from build123d import *

# Parameters (mm, degrees)
SKETCH35_R          = 1.5875
SKETCH35_R_2        = 55.372
BOSS_EXTRUDE5_DEPTH = 3.175


with BuildPart() as part:
    # Sketch35 → Boss-Extrude5 (new body)
    with BuildSketch(Plane(origin=(0, 0, 0), x_dir=(1, 0, 0), z_dir=(0, 1, 0))):
        with BuildLine():
            ThreePointArc((72.63160158, -196.735304264), (79.763343901, -189.694281524), (72.63160158, -182.653258784))
            ThreePointArc((72.63160158, -182.653258784), (71.923524594, -182.763416409), (71.274394231, -183.066957991))
            ThreePointArc((71.274394231, -183.066957991), (62.061766366, -186.749902585), (52.140854077, -186.639937081))
            ThreePointArc((52.140854077, -186.639937081), (49.212807322, -185.841233605), (46.400330688, -184.700461837))
            ThreePointArc((46.400330688, -184.700461837), (40.308522411, -162.14266409), (26.470306292, -143.315339746))
            ThreePointArc((26.470306292, -143.315339746), (2.051929923, -129.089326239), (-26.120702924, -126.866867398))
            ThreePointArc((-26.120702924, -126.866867398), (-27.858708089, -124.378751024), (-29.2889381, -121.701844758))
            ThreePointArc((-29.2889381, -121.701844758), (-31.603757208, -112.05414008), (-30.063154281, -102.252959759))
            ThreePointArc((-30.063154281, -102.252959759), (-29.911668214, -101.552560093), (-29.961834423, -100.837723697))
            ThreePointArc((-29.961834423, -100.837723697), (-38.413285984, -95.451564003), (-43.690813622, -103.971273609))
            ThreePointArc((-43.690813622, -103.971273609), (-43.425855926, -104.63708525), (-42.98547967, -105.202396203))
            ThreePointArc((-42.98547967, -105.202396203), (-37.34487163, -113.364511982), (-35.244469401, -123.061155914))
            ThreePointArc((-35.244469401, -123.061155914), (-35.371596014, -126.093518667), (-35.857931325, -129.089326239))
            ThreePointArc((-35.857931325, -129.089326239), (-74.114523813, -162.14266409), (-76.104068675, -212.661291576))
            ThreePointArc((-76.104068675, -212.661291576), (-78.143060244, -214.909379303), (-80.434594764, -216.899418143))
            ThreePointArc((-80.434594764, -216.899418143), (-89.325315633, -221.303016159), (-99.223576302, -221.982007162))
            ThreePointArc((-99.223576302, -221.982007162), (-99.940124308, -221.990172755), (-100.625875231, -222.198147255))
            ThreePointArc((-100.625875231, -222.198147255), (-103.996367762, -231.636236566), (-94.515904683, -234.885631829))
            ThreePointArc((-94.515904683, -234.885631829), (-93.925744965, -234.479160148), (-93.472600473, -233.924031523))
            ThreePointArc((-93.472600473, -233.924031523), (-86.770279347, -226.608603676), (-77.784133989, -222.403156653))
            ThreePointArc((-77.784133989, -222.403156653), (-74.799510568, -221.852331744), (-71.770594359, -221.659843715))
            ThreePointArc((-71.770594359, -221.659843715), (-52.467656797, -242.300414596), (-26.120702924, -252.52169565))
            ThreePointArc((-26.120702924, -252.52169565), (-2.772921395, -251.602203947), (18.661655395, -242.300414596))
            ThreePointArc((18.661655395, -242.300414596), (21.307097177, -243.788037808), (23.75715599, -245.579293472))
            ThreePointArc((23.75715599, -245.579293472), (30.028718121, -253.267212663), (32.893255611, -262.766213559))
            ThreePointArc((32.893255611, -262.766213559), (33.060663407, -263.462979195), (33.416017488, -264.085258231))
            ThreePointArc((33.416017488, -264.085258231), (43.367479341, -265.271073029), (44.425803982, -255.305246485))
            ThreePointArc((44.425803982, -255.305246485), (43.898200503, -254.82033176), (43.256155975, -254.502076287))
            ThreePointArc((43.256155975, -254.502076287), (34.632734421, -249.595632182), (28.533121278, -241.770588249))
            ThreePointArc((28.533121278, -241.770588249), (27.331965509, -238.983365642), (26.470306292, -236.073223302))
            ThreePointArc((26.470306292, -236.073223302), (40.308522411, -217.245898958), (46.400330688, -194.68810121))
            ThreePointArc((46.400330688, -194.68810121), (49.212807322, -193.547329442), (52.140854077, -192.748625967))
            ThreePointArc((52.140854077, -192.748625967), (62.061766366, -192.638660462), (71.274394231, -196.321605056))
            ThreePointArc((71.274394231, -196.321605056), (71.923524594, -196.625146639), (72.63160158, -196.735304264))
        make_face()
        with Locations(Location((72.72174416, -189.694281524, 0), (0, 0, 270))):
            Circle(SKETCH35_R, mode=Mode.SUBTRACT)
        with Locations(Location((-16.903000701, -189.694281524, 0), (0, 0, 270))):
            Circle(SKETCH35_R_2, mode=Mode.SUBTRACT)
        with Locations(Location((-97.652105615, -228.581000942, 0), (0, 0, 270))):
            Circle(SKETCH35_R, mode=Mode.SUBTRACT)
        with Locations(Location((-36.846382633, -102.316616136, 0), (0, 0, 270))):
            Circle(SKETCH35_R, mode=Mode.SUBTRACT)
        with Locations(Location((38.977113714, -259.765728664, 0), (0, 0, 270))):
            Circle(SKETCH35_R, mode=Mode.SUBTRACT)
    extrude(amount=BOSS_EXTRUDE5_DEPTH)


solid = part.part
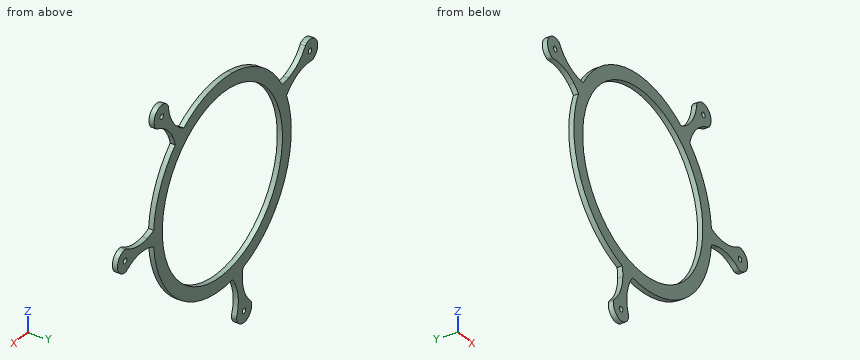
Build history of the part. All positions in model axes, mm. Round coordinates to 2 decimals unless told otherwise and drop trailing zeros. Order: outer loops, then holes, each group sorted by start corner. A loop starts at its lowest first (then second) coordinate and runs counter-clockwise, first axis right, second up. Notation, with made-up numbers: M 66,-26.75 L 115,-26.75 A9 cw 115,-14.75 Z; hole C 28.25,-9.75 d6. An arc over 180 degrees is marked long. Use CSV: the item, a comma, the result in double quotes. Start each with the question number.
(1) Cut at B-B on z = 179.5. List the corners of the cut face in (x, y) (1 decimal).
(2) Cut at C-C on y = 1. State how many separate pieces and enclosed holes the cut face has, then the cut area to 3 significant figures.
(3) Flat gauge pins, fed straight in: P1, Ø1, axis at x = 38.5, y = 2, coming from the -Z side; P2, Ø1.5, axis at y = 2, z = 166.5, coming from the +X side; P3, Ø1, axis at y = 1.5, z = 232.5, coming from the +X side. Where does each tip first touch, or does it go through?
(4) Cut at A-A on x = 8.5. List the corners of the cut face in (y, z) (3 decimals), then the cut area to 3 significant figures.
(5) Drill centre lines: probe 1 along X at (y, z) = (0.3, 190); probe 2 along X at (y, z) = (0.6, 195); probe 3 along Z at (x, y) = (34.5, 2.2). Where is each one in solid material? Low to high.
(6) Cut at D-D on z = 114. List the corners of the cut face in (x, y) (3 decimals).
Findings:
1,outline,"M -79.6,0 L -71.3,0 L -71.3,3.2 L -79.6,3.2 Z; M 37.5,0 L 45.8,0 L 45.8,3.2 L 37.5,3.2 Z"
2,separate pieces,"1"
2,enclosed holes,"5"
2,area,"4,110 mm^2"
3,P1,"stops at z = 157.79"
3,P2,"stops at x = 42.5"
3,P3,"stops at x = 30.45"
4,outline,"M 0,131.497 L 3.175,131.497 L 3.175,140.493 L 0,140.493 Z; M 0,238.895 L 3.175,238.895 L 3.175,247.892 L 0,247.892 Z"
4,area,"57.1 mm^2"
5,probe 1,"x = -80.4 to -72.27, 38.47 to 71.16, 74.28 to 79.76"
5,probe 2,"x = -80.18 to -72.02, 38.21 to 46.37, 68.99 to 77.35"
5,probe 3,"z = 152.41 to 169.11, 210.28 to 226.98, 249.48 to 265.2"
6,outline,"M -37.08,0 L -31.452,0 L -31.452,3.175 L -37.08,3.175 Z"
